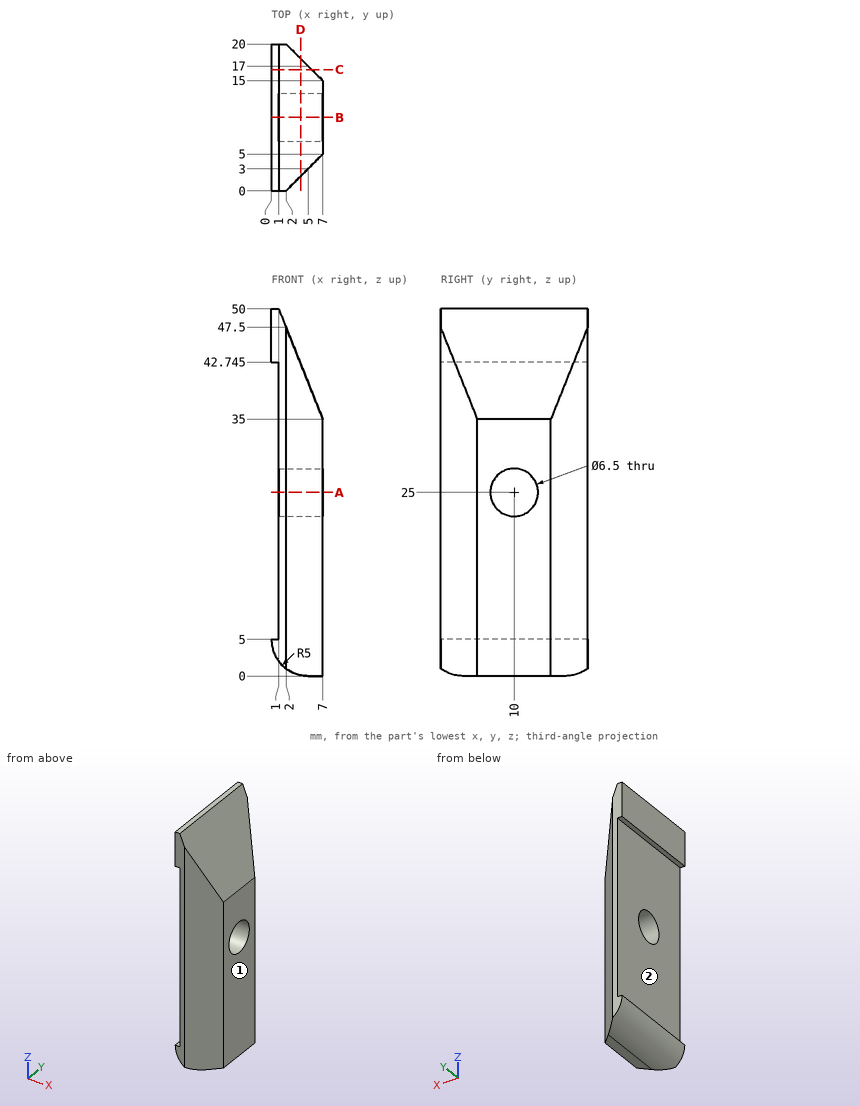
Check sheet for the drawn part. Datum: minimum x, y, z corner. Units: mm. A direction names the side the tool comes from. Round coordinates to 2 decimals unless told otherwise and drop trailing zeros. Loops run counter-clockwise (first coordinate to the right, second up) from the corner with the lowest first, then second, coordinate; pieces in that order, holes last. Notation, with made-up numbers: (45, 48) - (53, 48) arc R27 ccw to (53, 78) - close; hole circle Ø2 at (-34.75, 7.5). An arc over 180 degrees is marked (long way). Write each question's results on one line, items separated by ' | '. Start each with the question number.
Q1. Gauge pin test, flat ends, axial feed: P1, Ø2, axis at x = 6, y = 2.5, coming from the -Z side; P2, Ø2, axis at y = 2.5, z = 30.5, coming from the +X side; P3, Ø2, axis at x = 3, y = 15.5, coming from the -Z side; P4, Ø3, axis at y = 10.5, z = 10, coming from the -X side. Record the tip position at first contact, or that the pin passes through.
Q2. Cross-section at C-C on y = 16.5. Enter the section's corners in (x, z) (3 decimals), and give its area (3 significant figures).
Q3. Cross-section at B-B on y = 10. Enter the section's corners in (x, z) (3 decimals), and give its area (3 significant figures).
Q4. Thickness scan on line 1 (X direction, y = 14, z = 35); line 2 (X direction, y = 16, z = 45); line 3 (Z direction, x = 0.5, y = 11.5) (3 decimals). Record the ranges inside material, lowest first. Write a range as [from, to].
Q5. Access from +Z, -Z, +X, -X, +Y, -Y to the whole of each face (thin tool, end or side, straight path). Record for the marked faces 1 and 2.
Q6. Cross-section at D-D on x = 4. Enter the section's corners in (y, z).
Q7. Cross-section at A-A on z = 25. Enter the section's corners in (x, y), and give its area (3 significant figures).
Answers below:
1) P1: passes through | P2: stops at x = 5.5 | P3: stops at z = 0.1 | P4: stops at x = 1
2) outline: (0, 5) arc R5 ccw to (5, 0) - (5.5, 0) - (5.5, 38.75) - (1, 50) - (0, 50) - (0, 42.745) - (1, 42.745) - (1, 5) - close | area: 207 mm²
3) outline: (0, 5) arc R5 ccw to (5, 0) - (7, 0) - (7, 21.75) - (1, 21.75) - (1, 5) - close; (0, 42.745) - (1, 42.745) - (1, 28.25) - (7, 28.25) - (7, 35) - (1, 50) - (0, 50) - close | area: 223 mm²
4) line 1: x = [1, 7] | line 2: x = [0, 3] | line 3: z = [2.821, 5], [42.745, 50]
5) face 1: +Z, -Z, +X, +Y, -Y | face 2: -X, +Y, -Y
6) outline: (2, 0.1) - (18, 0.1) - (18, 42.5) - (2, 42.5) - close; hole circle Ø6.5 at (10, 25)
7) outline: (1, 0) - (2, 0) - (7, 5) - (7, 6.75) - (1, 6.75) - close; (1, 13.25) - (7, 13.25) - (7, 15) - (2, 20) - (1, 20) - close | area: 56.0 mm²
